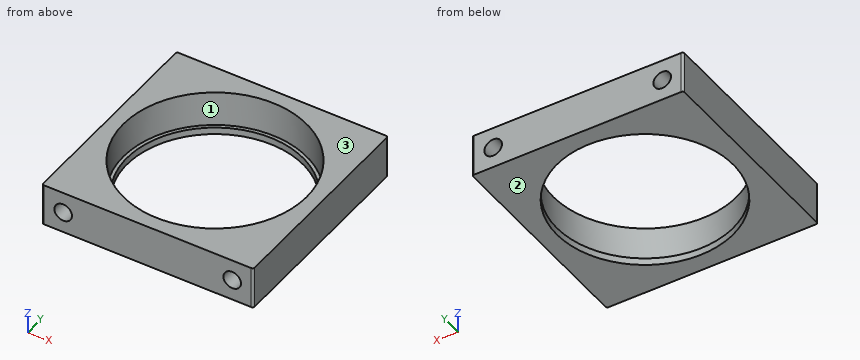
```python
from build123d import *

# Parameters (mm, degrees)
ESQUISSE1_W                                   = 30
ESQUISSE1_H                                   = 30
ESQUISSE1_R                                   = 12.5
BOSS_EXTRU_1_DEPTH                            = 6
ESQUISSE3_R                                   = 13
ENL_V_MAT_EXTRU_1_DEPTH                       = 5
TROU_POUR_TARAUDAGE_POUR_TROU_TARAUD_M3_D     = 2.5
TROU_POUR_TARAUDAGE_POUR_TROU_TARAUD_M3_DEPTH = 6
TROU_POUR_TARAUDAGE_POUR_TROU_TARAUD_M3_TIP   = 0.751075774
TROU_POUR_TARAUDAGE_POUR_TROU_TARAUD_2_D      = 2.5
TROU_POUR_TARAUDAGE_POUR_TROU_TARAUD_2_DEPTH  = 6
TROU_POUR_TARAUDAGE_POUR_TROU_TARAUD_2_TIP    = 0.751075774
CONG_1_R                                      = 0.3


with BuildPart() as part:
    # Esquisse1 → Boss.-Extru.1 (new body)
    with BuildSketch(Plane.XY):
        with Locations((15, 15)):
            Rectangle(ESQUISSE1_W, ESQUISSE1_H)
        with Locations((15, 15)):
            Circle(ESQUISSE1_R, mode=Mode.SUBTRACT)
    extrude(amount=BOSS_EXTRU_1_DEPTH)

    # Esquisse3 → Enlèv. mat.-Extru.1 (cut)
    with BuildSketch(Plane.XY.offset(6)):
        with Locations((15, 15)):
            Circle(ESQUISSE3_R)
    extrude(amount=-ENL_V_MAT_EXTRU_1_DEPTH, mode=Mode.SUBTRACT)

    # Trou pour taraudage pour trou taraud_ M3
    with Locations(Plane(origin=(0, 30, 0), x_dir=(1, 0, 0), z_dir=(0, 1, 0))):
        with Locations((3, -3), (27, -3)):
            Hole(TROU_POUR_TARAUDAGE_POUR_TROU_TARAUD_M3_D / 2, depth=TROU_POUR_TARAUDAGE_POUR_TROU_TARAUD_M3_DEPTH)
            with Locations((0, 0, -(TROU_POUR_TARAUDAGE_POUR_TROU_TARAUD_M3_DEPTH + TROU_POUR_TARAUDAGE_POUR_TROU_TARAUD_M3_TIP / 2))):  # 118° drill point
                Cone(0, TROU_POUR_TARAUDAGE_POUR_TROU_TARAUD_M3_D / 2, TROU_POUR_TARAUDAGE_POUR_TROU_TARAUD_M3_TIP, mode=Mode.SUBTRACT)

    # Trou pour taraudage pour trou taraud 2
    with Locations(Plane(origin=(0, 0, 0), x_dir=(-1, 0, 0), z_dir=(0, -1, 0))):
        with Locations((-3, -3), (-27, -3)):
            Hole(TROU_POUR_TARAUDAGE_POUR_TROU_TARAUD_2_D / 2, depth=TROU_POUR_TARAUDAGE_POUR_TROU_TARAUD_2_DEPTH)
            with Locations((0, 0, -(TROU_POUR_TARAUDAGE_POUR_TROU_TARAUD_2_DEPTH + TROU_POUR_TARAUDAGE_POUR_TROU_TARAUD_2_TIP / 2))):  # 118° drill point
                Cone(0, TROU_POUR_TARAUDAGE_POUR_TROU_TARAUD_2_D / 2, TROU_POUR_TARAUDAGE_POUR_TROU_TARAUD_2_TIP, mode=Mode.SUBTRACT)

    # Congé1
    cong_1_edges = [part.edges().sort_by_distance(p)[0] for p in [
        (0, 30, 3),
        (30, 30, 3),
        (30, 0, 3),
        (0, 0, 3),
    ]]
    fillet(cong_1_edges, radius=CONG_1_R)


solid = part.part
```
Input: part model. Units: mm. Frame: model coordinates. Face numbers are marked on the shaded views. Coordinates: 2 decimals unless noted, no trailing zeros. Write each loop counter-clockwise with the first axis right and the second up, starting at its lowest first coordinate (ties: lowest second). Pieces come first, ordered by that corner, then holes.
1) Mould query, pull axis Z, two halves, no side actions, for the marked faces 1, 2 and 3. Classes: pulls with the +Z half, pulls with the -Z half, needs draft (parallel to the pull), parting line crosses it, or undercut.
2) Section B-B on x = 6.75. Output: boundary loops of the cut face in (y, z), and give its area (3 significant figures).
3) Section D-D on y = 25. Output: boundary loops of the cut face in (x, z).
4) Material intervals for line 1 along Y through (x, z) = (15, 0.6); line 2 along Z through (x, y) = (27, 4.4); line 3 along X through (y, z) = (23.5, 3), sorted ascending.
5) Pin query (flat end, axial travel): pin 1 Ø8 at (x, y) = (9.5, 15) entering from +Z; pin 2 Ø3 at (x, z) = (3, 3) entering from +Y; pin 3 Ø2 at (x, z) = (3, 3) entering from -Y; pin 4 Ø1.5 at (x, z) = (27, 3) entering from +Y. Return the tip coordinate at first contact, or that it passes through.
6) Section C-C on z = 0.4. Output: boundary loops of the cut face in (x, y), and give its area (3 significant figures).
7) Section A-A on y = 15. Output: boundary loops of the cut face in (x, z), and give its area (3 significant figures).
Check result:
1. face 1: needs draft
1. face 2: pulls with the -Z half
1. face 3: pulls with the +Z half
2. outline: (0, 0) - (5.61, 0) - (5.61, 1) - (4.95, 1) - (4.95, 6) - (0, 6) - close; (24.39, 0) - (30, 0) - (30, 6) - (25.05, 6) - (25.05, 1) - (24.39, 1) - close
2. area: 60.8 mm2
3. outline: (0, 0) - (7.5, 0) - (7.5, 1) - (6.69, 1) - (6.69, 6) - (0, 6) - close; (22.5, 0) - (30, 0) - (30, 6) - (23.31, 6) - (23.31, 1) - (22.5, 1) - close; hole circle Ø2.5 at (3, 3); hole circle Ø2.5 at (27, 3)
4. line 1: y = 0 to 2.5, 27.5 to 30
4. line 2: z = 0 to 1.75, 4.25 to 6
4. line 3: x = 0 to 2.58, 3.42 to 5.16, 24.84 to 26.58, 27.42 to 30
5. pin 1: passes through
5. pin 2: stops at y = 30
5. pin 3: stops at y = 6.15
5. pin 4: stops at y = 23.7
6. outline: (0, 0.3) arc R0.3 ccw to (0.3, 0) - (29.7, 0) arc R0.3 ccw to (30, 0.3) - (30, 29.7) arc R0.3 ccw to (29.7, 30) - (0.3, 30) arc R0.3 ccw to (0, 29.7) - close; hole circle Ø25 at (15, 15)
6. area: 409 mm2
7. outline: (0, 0) - (2.5, 0) - (2.5, 1) - (2, 1) - (2, 6) - (0, 6) - close; (27.5, 0) - (30, 0) - (30, 6) - (28, 6) - (28, 1) - (27.5, 1) - close
7. area: 25.0 mm2
